from build123d import *

# Parameters (mm, degrees)
SKETCH1_R           = 2.159
BOSS_EXTRUDE1_DEPTH = 1.5875
FILLET1_R           = 9.525


with BuildPart() as part:
    # Sketch1 → Boss-Extrude1 (new, symmetric)
    with BuildSketch(Plane.XY):
        Polygon((0, 0), (69.85, 0), (69.85, 34.925), (34.925, 69.85), (0, 69.85), align=None)
        with Locations((50.825, 26.9625)):
            Circle(SKETCH1_R, mode=Mode.SUBTRACT)
        with Locations(Location((26.9625, 50.825, 0), (0, 0, 180))):
            Circle(SKETCH1_R, mode=Mode.SUBTRACT)
        with Locations((50.825, 7.9625)):
            Circle(SKETCH1_R, mode=Mode.SUBTRACT)
        with Locations(Location((7.9625, 50.825, 0), (0, 0, 180))):
            Circle(SKETCH1_R, mode=Mode.SUBTRACT)
        with Locations((41.325, 17.4625)):
            Circle(SKETCH1_R, mode=Mode.SUBTRACT)
        with Locations(Location((17.4625, 41.325, 0), (0, 0, 180))):
            Circle(SKETCH1_R, mode=Mode.SUBTRACT)
        with Locations((60.325, 17.4625)):
            Circle(SKETCH1_R, mode=Mode.SUBTRACT)
        with Locations(Location((17.4625, 60.325, 0), (0, 0, 180))):
            Circle(SKETCH1_R, mode=Mode.SUBTRACT)
    extrude(amount=BOSS_EXTRUDE1_DEPTH, both=True)

    # Fillet1
    fillet1_edges = [part.edges().sort_by_distance(p)[0] for p in [
        (0, 69.85, 0),
        (34.925, 69.85, 0),
        (69.85, 34.925, 0),
        (69.85, 0, 0),
        (0, 0, 0),
    ]]
    fillet(fillet1_edges, radius=FILLET1_R)


solid = part.part
Could you check a few things on this model? Use its own coordinates, in mm. Give positions to 0.01 mm unless a question says otherwise; leave off trailing zeros. Order: outer loops, then holes, each group sorted by start corner. A loop starts at its lowest first (then second) coordinate and runs counter-clockwise, first axis right, second up. Notation, with made-up numbers: (53.25, 44) - (98.25, 44) arc R18 cw to (98.25, 63) - close; hole circle Ø11 at (42.5, 35). An arc over 180 degrees is marked (long way). Return JSON: item names as keys, results as strings. Group by question number.
Q1. Suppose I cut it at D-D, the plane y = 65. Please give me the cut outline in (x, z) (1 decimal), and give its area (3 significant figures).
Q2. Thinking about a two-plate mould opening in Y: for faces 1 (the face through (69.105, 34.673, 0.022)), 2 (the face through (0, 35, 0)), 3 (the face through (17.744, 39.184, -0.022)), which applies, pulls with the +Y half, pulls with the -Y half, needs draft (parallel to the pull), parting line crosses it, or undercut?
Q3. Suppose I cut it at B-B, the plane z = 0. State how many separate pieces and enclosed holes the cut face has, and give its area (3 significant figures).
Q4. Will these pins go through, and if not, where does the flat tip stop? pin 1 Ø1 at (y, z) = (50.5, -1) entering from +X (3 decimals); pin 2 Ø5 at (x, y) = (7.96, 50.82) entering from -Z; pin 3 Ø4 at (x, y) = (60.32, 17.46) entering from +Z (3 decimals).
Q5. Please list where these lines run through material, in increasing order: line 1 along Y through (x, z) = (18, 0.3); line 2 along X through (y, z) = (18.5, 0.3); line 3 along X through (y, z) = (62, -1.1) (3 decimals). Write a range as [from, to].
Q6. Suppose I cut it at C-C, the plane x = 47. Please give me the cut outline in (y, z) (1 decimal), and give its area (3 significant figures).
Q7. Suppose I cut it at A-A, the plane y = 28. Please give me the cut outline in (x, z).
Resolved:
{
 "1": {"outline": "(1.2, -1.6) - (39.8, -1.6) - (39.8, 1.6) - (1.2, 1.6) - close", "area": "122 mm2"},
 "2": {"face 1": "pulls with the +Y half", "face 2": "needs draft", "face 3": "undercut"},
 "3": {"separate pieces": "1", "enclosed holes": "8", "area": "4,090 mm2"},
 "4": {"pin 1": "stops at x = 54.775", "pin 2": "stops at z = -1.59", "pin 3": "passes through"},
 "5": {"line 1": "y = [0, 39.23], [43.42, 58.23], [62.42, 69.85]", "line 2": "x = [0, 39.43], [43.22, 58.43], [62.22, 69.85]", "line 3": "x = [0.148, 16.1], [18.825, 42.775]"},
 "6": {"outline": "(0, -1.6) - (57.8, -1.6) - (57.8, 1.6) - (0, 1.6) - close", "area": "183 mm2"},
 "7": {"outline": "(0, -1.59) - (48.93, -1.59) - (48.93, 1.59) - (0, 1.59) - close; (52.72, -1.59) - (69.85, -1.59) - (69.85, 1.59) - (52.72, 1.59) - close"}
}
